from build123d import *

# Parameters (mm, degrees)
F0_W     = 1923
F0_H     = 600
F1_DEPTH = 19
F2_W     = 19
F2_H     = 541
F3_DEPTH = 120
F4_W     = 16
F4_H     = 581
F4_W_2   = 19
F5_DEPTH = 740
F6_W     = 1923
F6_H     = 120
F7_DEPTH = 19


with BuildPart() as f1:
    # F0 (on Top) → F1 (new body)
    with BuildSketch(Plane.XY):
        Rectangle(F0_W, F0_H)
    extrude(amount=F1_DEPTH)

    # F2 (on face) → F3 (join)
    with BuildSketch(Plane(origin=(0, 0, 0), x_dir=(1, 0, 0), z_dir=(0, 0, -1))):
        with Locations((-952, -29.5)):
            Rectangle(F2_W, F2_H)
        Polygon((-961.5, 260), (-961.5, 241), (-942.5, 241), (-423.5, 241), (-404.5, 241), (-385.5, 241), (-245.5, 241), (-226.5, 241), (-207.5, 241), (304.5, 241), (323.5, 241), (342.5, 241), (942.5, 241), (961.5, 241), (961.5, 260), align=None)
        with Locations((-414, -29.5)):
            Rectangle(F2_W, F2_H)
        with Locations((-395, -29.5)):
            Rectangle(F2_W, F2_H)
        with Locations((952, -29.5)):
            Rectangle(F2_W, F2_H)
        with Locations((-236, -29.5)):
            Rectangle(F2_W, F2_H)
        with Locations((333, -29.5)):
            Rectangle(F2_W, F2_H)
        with Locations((-217, -29.5)):
            Rectangle(F2_W, F2_H)
        with Locations((314, -29.5)):
            Rectangle(F2_W, F2_H)
    extrude(amount=F3_DEPTH)

    # F4 (on face) → F5 (join)
    with BuildSketch(Plane.XY.offset(19)):
        with Locations((-953.5, -9.5)):
            Rectangle(F4_W, F4_H)
        Polygon((-961.5, 300), (-961.5, 281), (-945.5, 281), (-427.5, 281), (-411.5, 281), (-392.5, 281), (342.5, 281), (361.5, 281), (377.5, 281), (945.5, 281), (961.5, 281), (961.5, 300), align=None)
        with Locations((-419.5, -9.5)):
            Rectangle(F4_W, F4_H)
        with Locations((-402, -9.5)):
            Rectangle(F4_W_2, F4_H)
        with Locations((953.5, -9.5)):
            Rectangle(F4_W, F4_H)
        with Locations((352, -9.5)):
            Rectangle(F4_W_2, F4_H)
        with Locations((369.5, -9.5)):
            Rectangle(F4_W, F4_H)
    extrude(amount=F5_DEPTH)

    # F6 (on face) → F7 (join)
    with BuildSketch(Plane.XY.offset(759)):
        with Locations((0, -240)):
            Rectangle(F6_W, F6_H)
        with Locations((0, 240)):
            Rectangle(F6_W, F6_H)
    extrude(amount=F7_DEPTH)


solid = f1.part
Geometry check sheet. Reference: the model listing, model coordinates, mm. A direction names the side the tool comes from. Coordinates: 2 decimals unless noted, no trailing zeros. Order: outer loops, then holes, each group sorted by start corner. A loop starts at its lowest first (then second) coordinate and runs counter-clockwise, first axis right, second up. Notation, with made-up numbers: (38, 28) -> (81, 28) arc R24 cw to (81, 62) -> close; hole circle Ø10 at (25, 36). An arc over 180 degrees is marked (long way). Use a Markdown table: item, result. Add a question column.
1. Set-up check for faces 1 (the face through (45, 33, 0)), 2 (the face through (-392.5, -14, 384)), 3 (the face through (13, -260, -59)): record each of +Z, -Z, +X, -X, +Y, -Y from which the full face is reachable in a straight line by a thin tool's end or side.
2. Cross-section at B-B (x = -305). Enter the section's corners in (y, z).
3. Material ranges on L1, parallel to X at y = 238, z = 579; L2, parallel to Z at x = 210, y = 253; L3, parallel to X at y = 247, z = -54, recorded low to high.
4. Mould release check, pull along Z, two halves, no side actions. Record for faces 4 (the face through (-961.5, -4, 323)), 5 (the face through (-30, -239, 759)), 6 (the face through (-316, 33, 0)): pulls with the +Z half, pulls with the -Z half, needs draft (parallel to the pull), parting line crosses it, or undercut.
5. Cross-section at A-A (y = 262). Give the number of separate pieces and of enclosed holes in the cut face, and give its area (3 significant figures).
6. Cross-section at C-C (z = 463.5). Enter the section's corners in (x, y), and give its area (3 significant figures).
7. Go/stop test with flat-tipped pins: pin 1 Ø6 at (x, z) = (-523.5, 196) entering from -Y; pin 2 Ø4 at (x, y) = (-652, 21.5) entering from -Z; pin 3 Ø2 at (x, y) = (-286, 56) entering from +Z. Record where each tip stops, or that it passes through.
Filled sheet:
| question | item | result |
|---|---|---|
| 1 | face 1 | -Z, +Y |
| 1 | face 2 | -Y |
| 1 | face 3 | -Z, +X, -X, -Y |
| 2 | outline | (-300, 0) -> (-260, 0) -> (-260, -120) -> (-241, -120) -> (-241, 0) -> (300, 0) -> (300, 778) -> (180, 778) -> (180, 759) -> (281, 759) -> (281, 19) -> (-300, 19) -> close; (-300, 759) -> (-180, 759) -> (-180, 778) -> (-300, 778) -> close |
| 3 | L1 | -961.5 to -945.5, -427.5 to -392.5, 342.5 to 377.5, 945.5 to 961.5 |
| 3 | L2 | 0 to 19, 759 to 778 |
| 3 | L3 | -961.5 to -942.5, -423.5 to -385.5, -245.5 to -207.5, 304.5 to 342.5, 942.5 to 961.5 |
| 4 | face 4 | needs draft |
| 4 | face 5 | undercut |
| 4 | face 6 | pulls with the -Z half |
| 5 | separate pieces | 1 |
| 5 | enclosed holes | 3 |
| 5 | area | 167,000 mm2 |
| 6 | outline | (-961.5, -300) -> (-945.5, -300) -> (-945.5, 281) -> (-427.5, 281) -> (-427.5, -300) -> (-392.5, -300) -> (-392.5, 281) -> (342.5, 281) -> (342.5, -300) -> (377.5, -300) -> (377.5, 281) -> (945.5, 281) -> (945.5, -300) -> (961.5, -300) -> (961.5, 300) -> (-961.5, 300) -> close |
| 6 | area | 95,800 mm2 |
| 7 | pin 1 | y = 281 |
| 7 | pin 2 | z = 0 |
| 7 | pin 3 | z = 19 |
